Can you work these out from the model? Positions are in its coordinate system, mm. Face numbers are marked on the shaded views. A direction names the side the tool comes from. Coordinates: 2 decimals unless noted, no trailing zeros. Order: outer loops, then holes, each group sorted by start corner. A loop starts at its lowest first (then second) coordinate and runs counter-clockwise, first axis right, second up. Notation, with made-up numbers: (-14, 46.25) -> (31, 46.25) arc R22 ccw to (31, 65.25) -> close; hole circle Ø6 at (3, -29.5). An arc over 180 degrees is marked (long way). Answer in a Markdown table with one row per item.
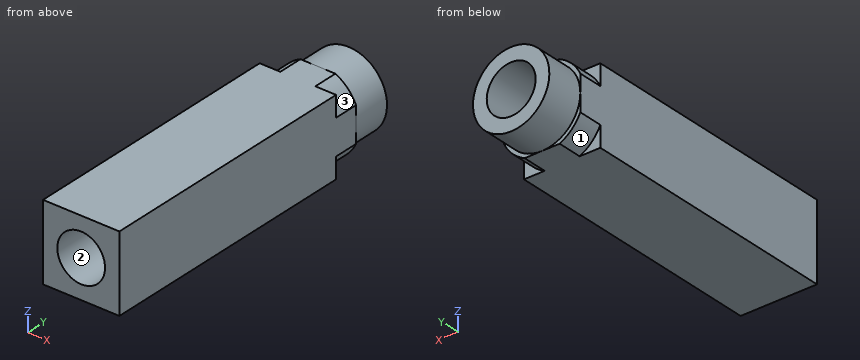
```python
from build123d import *

# Parameters (mm, degrees)
SKETCH1_W           = 6.35
SKETCH1_H           = 6.35
BOSS_EXTRUDE1_DEPTH = 22.225
SKETCH2_R           = 3.175
BOSS_EXTRUDE2_DEPTH = 27.45486
BOSS_EXTRUDE3_DEPTH = 2.05486
SKETCH5_R           = 1.984375
CUT_EXTRUDE1_DEPTH  = 12.7
SKETCH6_R           = 2.032
CUT_EXTRUDE2_DEPTH  = 12.7


with BuildPart() as part:
    # Sketch1 → Boss-Extrude1 (new body)
    with BuildSketch(Plane(origin=(0, 0, 0), x_dir=(1, 0, 0), z_dir=(0, 1, 0))):
        Rectangle(SKETCH1_W, SKETCH1_H)
    extrude(amount=BOSS_EXTRUDE1_DEPTH)

    # Sketch2 → Boss-Extrude2 (add)
    with BuildSketch(Plane.XZ):
        with Locations(Location((0, 0, 0), (0, 0, 270))):
            Circle(SKETCH2_R)
    extrude(amount=-BOSS_EXTRUDE2_DEPTH)

    # Sketch4 → Boss-Extrude3 (add)
    with BuildSketch(Plane(origin=(0, 24.27986, 0), x_dir=(1, 0, 0), z_dir=(0, 1, 0))):
        with BuildLine():
            Line((-3.175, 0), (-3.175, -1.454967783))
            ThreePointArc((-3.175, -1.454967783), (-2.469570433, -2.469570433), (-1.454967783, -3.175))
            Line((-1.454967783, -3.175), (0, -3.175))
            Line((0, -3.175), (1.454967783, -3.175))
            ThreePointArc((1.454967783, -3.175), (2.469570433, -2.469570433), (3.175, -1.454967783))
            Line((3.175, -1.454967783), (3.175, 0))
            Line((3.175, 0), (3.175, 1.454967783))
            ThreePointArc((3.175, 1.454967783), (2.469570433, 2.469570433), (1.454967783, 3.175))
            Line((1.454967783, 3.175), (0, 3.175))
            Line((0, 3.175), (-1.454967783, 3.175))
            ThreePointArc((-1.454967783, 3.175), (-2.469570433, 2.469570433), (-3.175, 1.454967783))
            Line((-3.175, 1.454967783), (-3.175, 0))
        make_face()
    extrude(amount=-BOSS_EXTRUDE3_DEPTH)

    # Sketch5 → Cut-Extrude1 (cut)
    with BuildSketch(Plane.XZ):
        with Locations(Location((0, 0, 0), (0, 0, 270))):
            Circle(SKETCH5_R)
    extrude(amount=-CUT_EXTRUDE1_DEPTH, mode=Mode.SUBTRACT)

    # Sketch6 → Cut-Extrude2 (cut)
    with BuildSketch(Plane(origin=(0, 27.45486, 0), x_dir=(1, 0, 0), z_dir=(0, 1, 0))):
        with Locations(Location((0, 0, 0), (0, 0, 270))):
            Circle(SKETCH6_R)
    extrude(amount=-CUT_EXTRUDE2_DEPTH, mode=Mode.SUBTRACT)


solid = part.part
```
(1) Will these pins go through, and if not, where does the flat tip stop? pin 1 Ø3 at (x, z) = (0, 0) entering from -Y; pin 2 Ø2 at (x, z) = (0, -0.5) entering from +Y.
Response values:
| item | result |
|---|---|
| pin 1 | y = 12.7 |
| pin 2 | y = 14.75 |
(2) I need wall thicknesses on line 1 (X direction, y = 20, z = 0) (3 decimals); line 2 (Z direction, x = 1.5, y = 5.5) (3 decimals); line 3 (X direction, y = 3.25, z = 0.5) (3 decimals). Which ranges of each line are inside material? Lowest first, please. Write a range as [from, to].
Response values:
| item | result |
|---|---|
| line 1 | [-3.175, -2.032], [2.032, 3.175] |
| line 2 | [-3.175, -1.299], [1.299, 3.175] |
| line 3 | [-3.175, -1.92], [1.92, 3.175] |
(3) Suppose I cut it at C-C (x = 1.75). Please give me the cut outline in (y, z) (3 decimals), and give its area (3 significant figures).
Response values:
| item | result |
|---|---|
| outline | (0, -3.175) -> (22.225, -3.175) -> (22.225, -3.022) -> (24.28, -3.022) -> (24.28, -2.649) -> (27.455, -2.649) -> (27.455, -1.033) -> (14.755, -1.033) -> (14.755, 1.033) -> (27.455, 1.033) -> (27.455, 2.649) -> (24.28, 2.649) -> (24.28, 3.022) -> (22.225, 3.022) -> (22.225, 3.175) -> (0, 3.175) -> (0, 0.936) -> (12.7, 0.936) -> (12.7, -0.936) -> (0, -0.936) -> close |
| area | 120 mm2 |
(4) Suppose I cut it at D-D (y = 17.25). Please give me the cut outline in (x, z) (3 decimals).
Response values:
| item | result |
|---|---|
| outline | (-3.175, -3.175) -> (3.175, -3.175) -> (3.175, 3.175) -> (-3.175, 3.175) -> close; hole circle Ø4.064 at (0, 0) |
(5) On a 3-axis mill with a long thin cutter (end or side, diameter ignored), from which of +Z, -Z, +X, -X, +Y, -Y can I reach the whole of each face in a straight line? I mean the marked faces 1, 2 and 3. Say none if no direction works.
Response values:
| item | result |
|---|---|
| face 1 | -Z, -X, +Y |
| face 2 | -Y |
| face 3 | +Z, +X, +Y |
(6) Suppose I cut it at B-B (z = -0.5). Please give me the cut outline in (x, y) (3 decimals).
Response values:
| item | result |
|---|---|
| outline | (-3.175, 0) -> (-1.92, 0) -> (-1.92, 12.7) -> (1.92, 12.7) -> (1.92, 0) -> (3.175, 0) -> (3.175, 24.28) -> (3.135, 24.28) -> (3.135, 27.455) -> (1.97, 27.455) -> (1.97, 14.755) -> (-1.97, 14.755) -> (-1.97, 27.455) -> (-3.135, 27.455) -> (-3.135, 24.28) -> (-3.175, 24.28) -> close |
(7) Suppose I cut it at A-A (y = 7.5). Please give me the cut outline in (x, z) (3 decimals), and give its area (3 significant figures).
Response values:
| item | result |
|---|---|
| outline | (-3.175, -3.175) -> (3.175, -3.175) -> (3.175, 3.175) -> (-3.175, 3.175) -> close; hole circle Ø3.969 at (0, 0) |
| area | 28.0 mm2 |
